Geometry check sheet. Reference: the model listing, model coordinates, mm. Face numbers are marked on the shaded views. Round coordinates to 2 decimals unless told otherwise and drop trailing zeros. Order: outer loops, then holes, each group sorted by start corner. A loop starts at its lowest first (then second) coordinate and runs counter-clockwise, first axis right, second up. Notation, with made-up numbers: (83, -24) - (106, -24) arc R19 ccw to (106, 13) - close; hole circle Ø7 at (62, -2.5). An arc over 180 degrees is marked (long way). Return JSON: item names as keys, results as strings. Group by question number.
Q1. Sectioned sample at B-B, the plane z = 0. Record the cut outline in (x, y) (1 decimal), then the cut area to 3 significant figures.
Q2. Gauge pin test, flat ends, axial feed: pin 1 Ø1 at (x, y) = (3.5, 8.5) entering from +Z; pin 2 Ø5 at (x, y) = (1.5, 3.5) entering from +Z; pin 3 Ø3 at (x, z) = (2.19, -1.62) entering from +Y. Record the tip position at first contact, or that the pin passes through.
Q3. Material ranges on line 1 along Z through (x, y) = (0, 7); line 2 along Z through (x, y) = (1, 15.25); line 3 along X through (y, z) = (2.25, 4.25), recorded low to high.
Q4. Draft check along X on the marked faces 1, 2 and 3. Enter one of: pulls with the +X half, pulls with the -X half, needs draft (parallel to the pull), parting line crosses it, or undercut.
Q5. Sectioned sample at A-A, the plane x = 0. Record the cut outline in (y, z) (1 decimal).
Q6. Sectioned sample at C-C, the plane y = 12.5. Record the cut outline in (x, z).
Autodesk Inventor part; units mm, degrees
ref_plane "YZ Plane" through (0, 0, 0) normal (1, 0, 0) x (0, 1, 0)
ref_plane "XZ Plane" through (0, 0, 0) normal (0, 1, 0) x (-1, 0, 0)
ref_plane "XY Plane" through (0, 0, 0) normal (0, 0, 1) x (1, 0, 0)
sketch "Sketch1" plane through (0, 0, 0) normal (0, 1, 0) x (-1, 0, 0)
  circle A0 centre (0, 0) radius 5.842
  dimension "d0" = 11.684
extrude "Extrusion1" add sketch "Sketch1" along normal blind 20.32
shell "Shell1" thickness 1.0922 removed faces 1 at (-0.5241, 20.32, 1.3818)
fillet "Fillet1" radius 1.5875 1 edges at (5.842, 0, 0)
sketch "Sketch2" plane through (0, 0, 0) normal (0, -1, 0) x (1, 0, 0)
  circle A0 centre (2.1901, -1.6223) radius 0.9525
  point P0 (0, 0)
  dimension "d5" = 1.905
extrude "Extrusion2" cut sketch "Sketch2" against normal through all
properties part number "bottun tube" material "Glass"
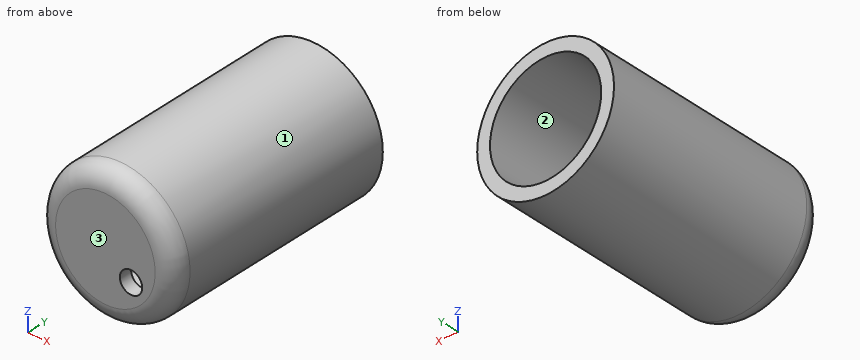
Reply:
{
 "1": {"outline": "(-5.8, 1.6) arc R1.6 ccw to (-4.3, 0) - (4.3, 0) arc R1.6 ccw to (5.8, 1.6) - (5.8, 20.3) - (4.7, 20.3) - (4.7, 1.1) - (-4.7, 1.1) - (-4.7, 20.3) - (-5.8, 20.3) - close", "area": "53.7 mm^2"},
 "2": {"pin 1": "z = 5.01", "pin 2": "z = 5.84", "pin 3": "y = 1.09"},
 "3": {"line 1": "-5.84 to -4.75, 4.75 to 5.84", "line 2": "-5.76 to -4.64, 4.64 to 5.76", "line 3": "-4.01 to -2.12, 2.12 to 4.01"},
 "4": {"face 1": "parting line crosses it", "face 2": "undercut", "face 3": "needs draft"},
 "5": {"outline": "(0, -4.3) arc R1.6 ccw to (1.6, -5.8) - (20.3, -5.8) - (20.3, -4.7) - (1.1, -4.7) - (1.1, 4.7) - (20.3, 4.7) - (20.3, 5.8) - (1.6, 5.8) arc R1.6 ccw to (0, 4.3) - close"},
 "6": {"outline": "circle Ø11.68 at (0, 0); hole circle Ø9.5 at (0, 0)"}
}
